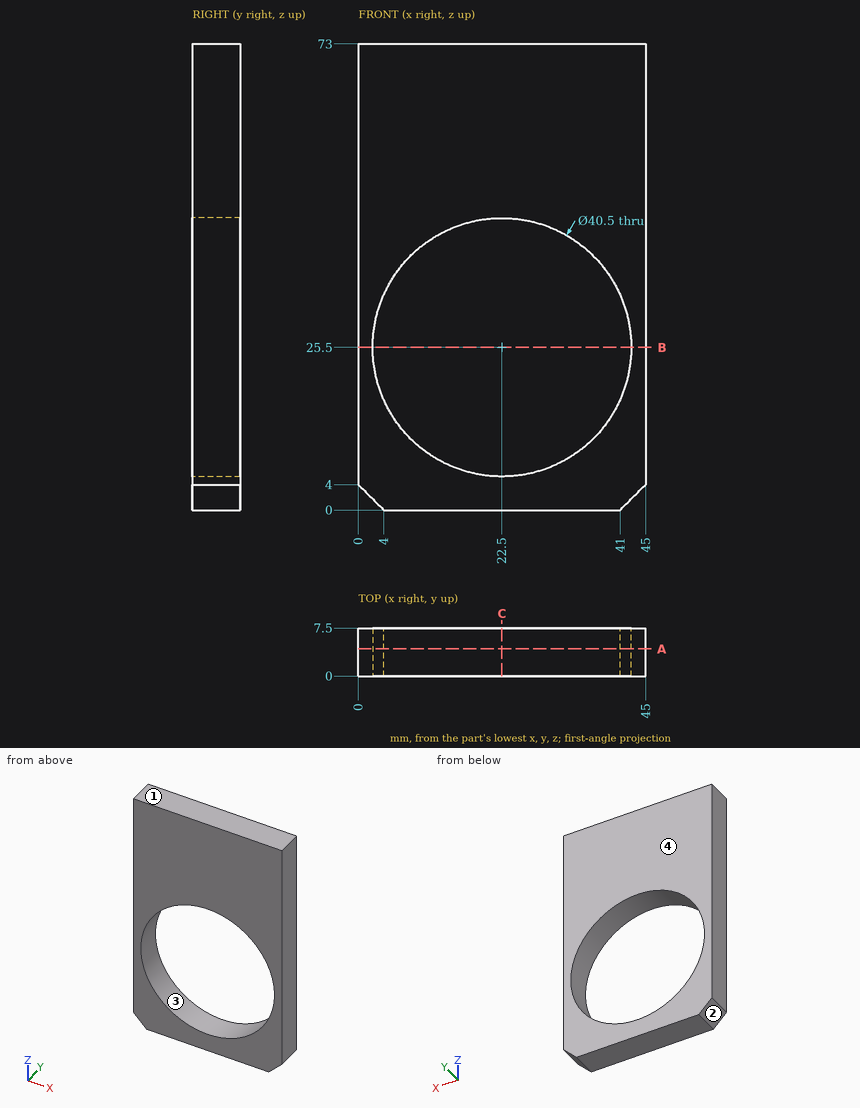
Print and shaded views of the part. All mm, measured from the part's lowest x, y and z. Give positions to 0.01 mm unless a question says otherwise; leave off trailing zeros. Write each loop counter-clockwise with the first axis right and the second up, starting at its lowest first coordinate (ties: lowest second). Pieces come first, ordered by that corner, then holes. Notation, with made-up numbers: (-18.5, 66) -> (34.5, 66) arc R17 ccw to (34.5, 90) -> close; hole circle Ø2 at (76, -1.75). An arc over 180 degrees is marked (long way). Write each question's results on one line, items separated by ' | '.
1. Cut at A-A, the plane y = 4.25. Write the cut outline in (x, z), then the cut area to 3 significant figures.
Geometry check:
outline: (0, 4) -> (4, 0) -> (41, 0) -> (45, 4) -> (45, 73) -> (0, 73) -> close; hole circle Ø40.5 at (22.5, 25.5) | area: 1,980 mm²
2. Cut at C-C, the plane x = 22.5. Write the cut outline in (y, z).
Geometry check:
outline: (0, 0) -> (7.5, 0) -> (7.5, 5.25) -> (0, 5.25) -> close; (0, 45.75) -> (7.5, 45.75) -> (7.5, 73) -> (0, 73) -> close
3. Two-plate mould, pull along Z, no slides. Class the marked faces 1, 2, 3 and 4: pulls with the +Z half, pulls with the -Z half, needs draft (parallel to the pull), parting line crosses it, or undercut.
Geometry check:
face 1: pulls with the +Z half | face 2: pulls with the -Z half | face 3: undercut | face 4: needs draft
4. Cut at B-B, the plane z = 25.5. Write the cut outline in (x, y).
Geometry check:
outline: (0, 0) -> (2.25, 0) -> (2.25, 7.5) -> (0, 7.5) -> close; (42.75, 0) -> (45, 0) -> (45, 7.5) -> (42.75, 7.5) -> close
5. Wall check: probe 1 along Z at (x, y) = (22.5, 5); probe 2 along X at (y, z) = (1.5, 25.5); probe 3 along Z at (x, y) = (15.5, 5.75). Give the ranges that are in metal, low to high. Write a range as [from, to].
Geometry check:
probe 1: [0, 5.25], [45.75, 73] | probe 2: [0, 2.25], [42.75, 45] | probe 3: [0, 6.5], [44.5, 73]
